The listing builds one solid part. Answer for the finished solid, in the listing's coordinates (mm). A direction names the side the tool comes from. Give positions to 0.01 mm unless a question says otherwise; leave off trailing zeros. Order: outer loops, then holes, each group sorted by start corner. A loop starts at its lowest first (then second) coordinate and runs counter-clockwise, first axis right, second up. Notation, with made-up numbers: (26, 54.25) - (81, 54.25) arc R27 cw to (81, 74.25) - close; hole circle Ø6 at (36, 77.25). An arc over 180 degrees is marked (long way). Answer as a JSON object with one key per item and string values. Group by question number.
Q1. For faces 4 (the face through (90.349, -0.258, -0.133)), 5 (the face through (121.2, -12.7, 9.525)), 6 (the face through (-132.08, -9, 0)), determine the directions among +Z, -Z, +X, -X, +Y, -Y from which every point of the face is accessible in a straight line to the end or side of a thin tool.
Q2. A cutting plane is placed at B-B, the plane x = -50.5. Give the vertices of the cut face in (y, z) (3 decimals), and give its area (3 significant figures).
Q3. The mould has two halves that part along X. Classify faces 1 (the face through (-120.1, -12.7, -9.525)), 2 (the face through (134.62, -9, 7)), 3 (the face through (118, -9, 11.112)): released by +X, released by -X, zero draft, split by the parting line, or undercut.
Q4. A cutting plane is placed at A-A, the plane x = 120.65. Give the vertices of the cut face in (y, z) (1 decimal), and give its area (3 significant figures).
Q5. Given pin 1 (5.5 mm diameter, centred on x = -81.28, y = -5.08, fed in from +Z) (3 decimals); pin 2 (2 mm diameter, centred on x = -81.28, y = -25.4, fed in from -Z); pin 3 (1 mm diameter, centred on x = -60.5, y = 4.5, fed in from -Z) (3 decimals); pin 4 (5 mm diameter, centred on y = 2, z = -0.5, fed in from +X), each flat-ended and moving along its own axis, determine where each tip first touches the part or whether it passes through.
Q6. Consider line 1 (X direction, y = -10, z = -4.5); line 2 (Y direction, x = 81.28, z = -4.5); line 3 (X direction, y = -4, z = -4.5). Determine where each line is inside the solid, lowest interval first.
from build123d import *

# Parameters (mm, degrees)
BOSS_EXTRUDE1_DEPTH      = 9.525
BOSS_EXTRUDE1_DEPTH_BACK = 9.525
SKETCH1_R                = 1.7
SKETCH2_W                = 2.54
SKETCH2_H                = 5.08
CUT_EXTRUDE1_DEPTH       = 27.686
BOSS_EXTRUDE2_DEPTH      = 1.5875


with BuildPart() as part:
    # Sketch1 → Boss-Extrude1 (new, two sides: drawn at the far end of the back side and taken through both)
    with BuildSketch(Plane.XY.offset(-BOSS_EXTRUDE1_DEPTH_BACK)):
        with BuildLine():
            Line((-109.22, 0), (-134.62, 0))
            Line((-134.62, 0), (-134.62, -17.78))
            Line((-134.62, -17.78), (-127, -17.78))
            ThreePointArc((-127, -17.78), (-120.65, -11.43), (-114.3, -17.78))
            Line((-114.3, -17.78), (-109.22, -17.78))
            Line((-109.22, -17.78), (-101.6, -17.78))
            Line((-101.6, -17.78), (-101.6, -3.81))
            ThreePointArc((-101.6, -3.81), (-100.112102448, -0.217897552), (-96.52, 1.27))
            Line((-96.52, 1.27), (-93.98, 1.27))
            ThreePointArc((-93.98, 1.27), (-90.387897552, -0.217897552), (-88.9, -3.81))
            Line((-88.9, -3.81), (-88.9, -17.78))
            Line((-88.9, -17.78), (-88.9, -27.94))
            Line((-88.9, -27.94), (88.9, -27.94))
            Line((88.9, -27.94), (88.9, -17.78))
            Line((88.9, -17.78), (88.9, -3.81))
            ThreePointArc((88.9, -3.81), (90.387897552, -0.217897552), (93.98, 1.27))
            Line((93.98, 1.27), (96.52, 1.27))
            ThreePointArc((96.52, 1.27), (100.112102448, -0.217897552), (101.6, -3.81))
            Line((101.6, -3.81), (101.6, -17.78))
            Line((101.6, -17.78), (109.22, -17.78))
            Line((109.22, -17.78), (114.3, -17.78))
            ThreePointArc((114.3, -17.78), (120.65, -11.43), (127, -17.78))
            Line((127, -17.78), (134.62, -17.78))
            Line((134.62, -17.78), (134.62, 0))
            Line((134.62, 0), (109.22, 0))
            Line((109.22, 0), (109.22, 17.78))
            Line((109.22, 17.78), (-109.22, 17.78))
            Line((-109.22, 17.78), (-109.22, 0))
        make_face()
        with Locations((-81.28, -25.4)):
            Circle(SKETCH1_R, mode=Mode.SUBTRACT)
        with Locations((-81.28, -5.08)):
            Circle(SKETCH1_R, mode=Mode.SUBTRACT)
        with Locations((81.28, -25.4)):
            Circle(SKETCH1_R, mode=Mode.SUBTRACT)
        with Locations((81.28, -5.08)):
            Circle(SKETCH1_R, mode=Mode.SUBTRACT)
    extrude(amount=BOSS_EXTRUDE1_DEPTH + BOSS_EXTRUDE1_DEPTH_BACK)

    # Sketch2 → Cut-Extrude1 (cut)
    with BuildSketch(Plane(origin=(0, 0, 0), x_dir=(1, 0, 0), z_dir=(0, 1, 0))):
        with Locations((-110.49, 0)):
            Rectangle(SKETCH2_W, SKETCH2_H)
        with Locations((-133.35, 0)):
            Rectangle(SKETCH2_W, SKETCH2_H)
        with Locations((133.35, 0)):
            Rectangle(SKETCH2_W, SKETCH2_H)
        with Locations((110.49, 0)):
            Rectangle(SKETCH2_W, SKETCH2_H)
    extrude(amount=-CUT_EXTRUDE1_DEPTH, mode=Mode.SUBTRACT)

    # Sketch3 → Boss-Extrude2 (add)
    with BuildSketch(Plane.XY.offset(9.525)):
        with BuildLine():
            Line((-134.62, 0), (-101.6, 0))
            Line((-101.6, 0), (-101.6, -17.78))
            Line((-101.6, -17.78), (-115.824, -17.78))
            ThreePointArc((-115.824, -17.78), (-120.65, -12.954), (-125.476, -17.78))
            Line((-125.476, -17.78), (-134.62, -17.78))
            Line((-134.62, -17.78), (-134.62, 0))
        make_face()
        with BuildLine():
            Line((134.62, -17.78), (125.476, -17.78))
            ThreePointArc((125.476, -17.78), (120.65, -12.954), (115.824, -17.78))
            Line((115.824, -17.78), (101.6, -17.78))
            Line((101.6, -17.78), (101.6, 0))
            Line((101.6, 0), (134.62, 0))
            Line((134.62, 0), (134.62, -17.78))
        make_face()
    boss_extrude2 = extrude(amount=BOSS_EXTRUDE2_DEPTH)

    # Mirror1: Boss-Extrude2 across plane
    add(boss_extrude2.mirror(Plane.XY))


solid = part.part
Reply:
{
 "1": {"face 4": "+Z, -Z, -Y", "face 5": "-Y", "face 6": "-X, +Y, -Y"},
 "2": {"outline": "(-27.94, -9.525) - (17.78, -9.525) - (17.78, 9.525) - (-27.94, 9.525) - close", "area": "871 mm^2"},
 "3": {"face 1": "undercut", "face 2": "released by +X", "face 3": "zero draft"},
 "4": {"outline": "(-13, -11.1) - (0, -11.1) - (0, 11.1) - (-13, 11.1) - (-13, 9.5) - (-11.4, 9.5) - (-11.4, -9.5) - (-13, -9.5) - close", "area": "259 mm^2"},
 "5": {"pin 1": "stops at z = 9.525", "pin 2": "passes through", "pin 3": "stops at z = -9.525", "pin 4": "stops at x = 132.08"},
 "6": {"line 1": "x = -134.62 to -101.6, -88.9 to 88.9, 101.6 to 134.62", "line 2": "y = -27.94 to -27.1, -23.7 to -6.78, -3.38 to 17.78", "line 3": "x = -134.62 to -101.6, -88.9 to -82.59, -79.97 to 79.97, 82.59 to 88.9, 101.6 to 134.62"}
}
